Source: CAD feature listing. Evaluate the final solid. Frame: model axes, mm. A direction names the side the tool comes from. Round coordinates to 2 decimals unless told otherwise and drop trailing zeros. Write each loop counter-clockwise with the first axis right and the second up, starting at its lowest first coordinate (ties: lowest second). Pieces come first, ordered by that corner, then holes. Notation, with made-up numbers: (38, -36.75) -> (54, -36.75) arc R21 cw to (54, -16.75) -> close; hole circle Ø5 at (-5, -4). An arc over 180 degrees is marked (long way). Put each result on its own line as item: value.
```python
from build123d import *

# Parameters (mm, degrees)
SKETCH1_R           = 11.1010859
SKETCH1_RX          = 11.1010859
SKETCH1_RY          = 7.064327391
BOSS_EXTRUDE1_DEPTH = 3


with BuildPart() as part:
    # Sketch1 → Boss-Extrude1 (new body)
    with BuildSketch(Plane.XY):
        with BuildLine():
            Line((-17.894214973, -7.255421854), (1.504545567, -14.356753838))
            ThreePointArc((1.504545567, -14.356753838), (3.673142738, -14.941061094), (5.91044133, -15.137844409))
            Line((5.91044133, -15.137844409), (28.826197236, -15.137844409))
            Line((28.826197236, -15.137844409), (46.358712744, -15.137844409))
            ThreePointArc((46.358712744, -15.137844409), (46.404537835, -14.634718136), (46.449065208, -14.131475353))
            ThreePointArc((46.449065208, -14.131475353), (45.733406698, -13.729506595), (45.553147083, -12.928724192))
            ThreePointArc((45.553147083, -12.928724192), (45.913364237, -12.337750174), (46.569590651, -12.117810222))
            ThreePointArc((46.569590651, -12.117810222), (47.144860113, 2.882189778), (46.569590651, 17.882189778))
            ThreePointArc((46.569590651, 17.882189778), (45.913364237, 18.102129729), (45.553147083, 18.693103748))
            ThreePointArc((45.553147083, 18.693103748), (45.733406698, 19.49388615), (46.449065208, 19.895854908))
            ThreePointArc((46.449065208, 19.895854908), (46.404537835, 20.399097691), (46.358712744, 20.902223964))
            Line((46.358712744, 20.902223964), (28.826197236, 20.902223964))
            Line((28.826197236, 20.902223964), (5.91044133, 20.902223964))
            ThreePointArc((5.91044133, 20.902223964), (3.673142738, 20.70544065), (1.504545567, 20.121133393))
            Line((1.504545567, 20.121133393), (-17.894214973, 13.019801409))
            ThreePointArc((-17.894214973, 13.019801409), (-21.907637047, 11.625593721), (-25.965065064, 10.365177235))
            ThreePointArc((-25.965065064, 10.365177235), (-32.222134734, 2.882189778), (-25.965065064, -4.60079768))
            ThreePointArc((-25.965065064, -4.60079768), (-21.907637047, -5.861214166), (-17.894214973, -7.255421854))
        make_face()
        with Locations((-0.54553615, 2.882189778)):
            Circle(SKETCH1_R, mode=Mode.SUBTRACT)
        with Locations(Location((19.45446385, 2.882189778), (0, 0, -90))):
            Ellipse(SKETCH1_RX, SKETCH1_RY, mode=Mode.SUBTRACT)
        with BuildLine():
            Line((-16.54553615, 0.106918303), (-24.619053168, 0.106918303))
            ThreePointArc((-24.619053168, 0.106918303), (-27.394324643, 2.882189778), (-24.619053168, 5.657461252))
            Line((-24.619053168, 5.657461252), (-16.54553615, 5.657461252))
            ThreePointArc((-16.54553615, 5.657461252), (-13.770264675, 2.882189778), (-16.54553615, 0.106918303))
        make_face(mode=Mode.SUBTRACT)
    extrude(amount=BOSS_EXTRUDE1_DEPTH)


solid = part.part
```
Q1. Material intervals for line 1 (X direction, y = -4, z = 0.75); line 2 (X direction, y = -2, z = 2); line 3 (X direction, y = 5, z = 1.3), sorted ascending. Write a range as [from, to].
Ans:
line 1: x = [-27.85, -9.26], [8.16, 13.91], [25, 47.02]
line 2: x = [-30.45, -10.52], [9.42, 13.11], [25.8, 47.08]
line 3: x = [-31.92, -26.41], [-14.75, -11.44], [10.35, 12.52], [26.39, 47.13]
Q2. Draft query along Y for faces 1 (the flat face through (26, -15.138, 1)), 2 (the cylindrical face through (-27.394, 2.821, 1.479)), 3 (the flat face through (-8.06, 16.62, 1.48)). Return one class per face: +Y half, -Y half, draft (parallel to the pull), parting line (faces both ways), or undercut.
Ans:
face 1: -Y half
face 2: undercut
face 3: +Y half
Q3. Reachability of faces 4 (the cylindrical face through (-21.851, 11.644, 1.479)), 5 (the flat face through (-21, 0.107, 1)) from +Z, -Z, +X, -X, +Y, -Y: full face, straight path, thin tool, end or side. Return the list, or none.
Ans:
face 4: +Z, -Z, -X, +Y
face 5: +Z, -Z
Q4. Cut plane D-D on x = -8. Output: boundary loops of the cut face in (y, z).
Ans:
outline: (-10.88, 0) -> (-5.34, 0) -> (-5.34, 3) -> (-10.88, 3) -> close; (11.11, 0) -> (16.64, 0) -> (16.64, 3) -> (11.11, 3) -> close
Q5. Pin query (flat end, axial travel): pin 1 (1.5 mm diameter, centred on y = -6, z = 2, fed in from +X); pin 2 (0.9 mm diameter, centred on x = -22.5, z = 2, fed in from -Y). Return the tip coordinate at first contact, or that it passes through.
Ans:
pin 1: stops at x = 46.98
pin 2: stops at y = -5.81
Q6. Cut plane B-B on y = -2. Give the number of separate pieces and of enclosed holes in the cut face, and give its area (3 significant figures).
Ans:
separate pieces: 3
enclosed holes: 0
area: 135 mm^2
Q7. Cut plane A-A on x = -19. Output: boundary loops of the cut face in (y, z), and give its area (3 significant figures).
Ans:
outline: (-6.86, 0) -> (0.11, 0) -> (0.11, 3) -> (-6.86, 3) -> close; (5.66, 0) -> (12.62, 0) -> (12.62, 3) -> (5.66, 3) -> close
area: 41.8 mm^2
